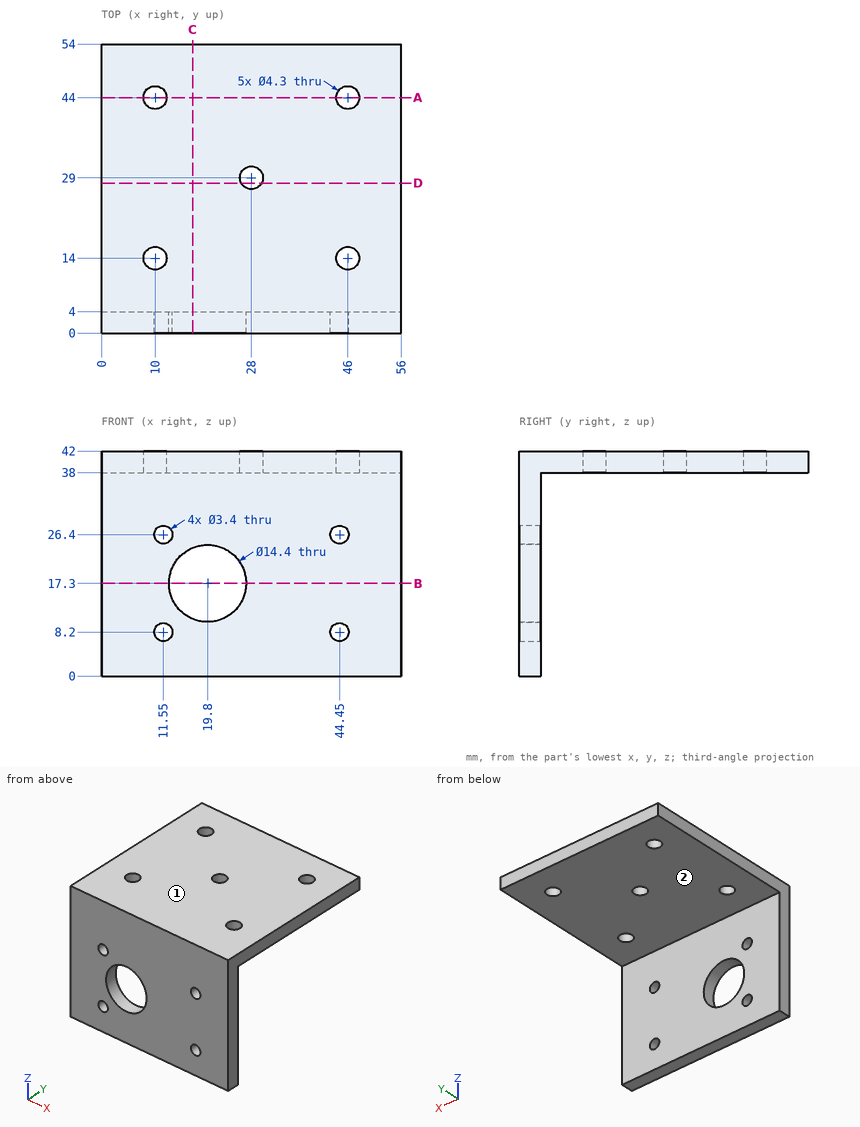
Geometry check sheet. Reference: drawing and pictorial views, mm from the part's lowest x, y, z. A direction names the side the tool comes from. Give positions to 0.01 mm unless a question says otherwise; leave off trailing zeros. Loops run counter-clockwise (first coordinate to the right, second up) from the corner with the lowest first, then second, coordinate; pieces in that order, holes last.
1. Go/stop test with flat-tipped pins: pin 1 Ø4 at (y, z) = (44, 35) entering from -X; pin 2 Ø25 at (x, y) = (28, 24) entering from -Z; pin 3 Ø4 at (x, z) = (44.45, 26.4) entering from +Y. Record where each tip stops, or that it passes through.
2. Section check A-A, the plane y = 44. Enter the section's corners in (x, z), then the cut area to 3 significant figures.
3. Thickness scan on line 1 (Y direction, x = 10, z = 40.25); line 2 (Y direction, x = 28, z = 40.75); line 3 (X direction, y = 2.8, z = 17.3). Record the ranges inside material, lowest first.
4. Section check C-C, the plane x = 17. Enter the section's corners in (y, z).
5. Set-up check for the marked faces 1 and 2: record each of +Z, -Z, +X, -X, +Y, -Y from which the full face is reachable in a straight line by a thin tool's end or side.
6. Section check D-D, the plane y = 28. Enter the section's corners in (x, z).
7. Section check B-B, the plane z = 17.3. Enter the section's corners in (x, y).
Geometry says:
1. pin 1: passes through
1. pin 2: stops at z = 38
1. pin 3: stops at y = 4
2. outline: (0, 38) - (7.85, 38) - (7.85, 42) - (0, 42) - close; (12.15, 38) - (43.85, 38) - (43.85, 42) - (12.15, 42) - close; (48.15, 38) - (56, 38) - (56, 42) - (48.15, 42) - close
2. area: 190 mm2
3. line 1: y = 0 to 11.85, 16.15 to 41.85, 46.15 to 54
3. line 2: y = 0 to 26.85, 31.15 to 54
3. line 3: x = 0 to 12.6, 27 to 56
4. outline: (0, 0) - (4, 0) - (4, 10.67) - (0, 10.67) - close; (0, 23.93) - (4, 23.93) - (4, 38) - (54, 38) - (54, 42) - (0, 42) - close
5. face 1: +Z, +X, -X, +Y, -Y
5. face 2: -Z, +X, -X, +Y
6. outline: (0, 38) - (26.1, 38) - (26.1, 42) - (0, 42) - close; (29.9, 38) - (56, 38) - (56, 42) - (29.9, 42) - close
7. outline: (0, 0) - (12.6, 0) - (12.6, 4) - (0, 4) - close; (27, 0) - (56, 0) - (56, 4) - (27, 4) - close
